Work out the finished part from the listing and answer in its coordinate system (mm). A direction names the side the tool comes from. Give positions to 0.01 mm unless a question says otherwise; leave off trailing zeros. Loops run counter-clockwise (first coordinate to the right, second up) from the corner with the lowest first, then second, coordinate; pieces in that order, holes last. Notation, with made-up numbers: (55, 26.5) - (71, 26.5) arc R26 cw to (71, 51.5) - close; hole circle Ø6 at (-35, -17). An arc over 180 degrees is marked (long way). Use one line per item in the form item = value. Start each with the question number.
Autodesk Inventor part; units mm, degrees
ref_plane "YZ Plane" through (0, 0, 0) normal (1, 0, 0) x (0, 1, 0)
ref_plane "XZ Plane" through (0, 0, 0) normal (0, 1, 0) x (-1, 0, 0)
ref_plane "XY Plane" through (0, 0, 0) normal (0, 0, 1) x (1, 0, 0)
sketch "Sketch1" plane through (0, 0, 0) normal (0, 1, 0) x (-1, 0, 0)
  circle A0 centre (0, 0) radius 21.5
  dimension "d0" = 43
extrude "Extrusion1" add sketch "Sketch1" along normal blind 68
sketch "Sketch2" plane through (0, 68, 0) normal (0, 1, 0) x (1, 0, 0)
  circle A0 centre (0, 0) radius 7.5
  dimension "d3" = 15
extrude "Extrusion2" add sketch "Sketch2" along normal blind 54
sketch "Sketch3" plane through (0, 0, 0) normal (0, -1, 0) x (1, 0, 0)
  line L0 (-15, 5) -> (-10, 5)
  line L1 (-10, 5) -> (-10, -5)
  line L2 (-10, -5) -> (-15, -5)
  line L3 (-15, -5) -> (-15, 5)
  line L4 (10, 5) -> (15, 5)
  line L5 (15, 5) -> (15, -5)
  line L6 (15, -5) -> (10, -5)
  line L7 (10, -5) -> (10, 5)
  line L8 (0, 0) -> (-29.5746, 0)
  circle A0 centre (0, 0) radius 7.5
  line L9 (0, 0) -> (0, 33.0968)
  dimension "d6" = 10
  dimension "d7" = 5
  dimension "d8" = 20
extrude "Extrusion3" add sketch "Sketch3" along normal blind 15 contours L0 L1 L8 L3 | L8 L1 L2 L3 | L4 L5 L6 L7
properties part number "Dremel motor"
1) A cutting plane is placed at B-B (z = 0). Give the vertices of the cut face in (x, y), plus the area to 3 significant figures.
2) A cutting plane is placed at D-D (x = 5.5). Give the vertices of the cut face in (y, z), plus the area to 3 significant figures.
3) Find the intervals of material crossed by probe 1 along X at (y, z) = (-4, -2); probe 2 along Y at (x, z) = (-17, 9.5); probe 3 along Z at (x, y) = (14, -4), in increasing order.
4) A cutting plane is placed at A-A (x = 0). Give the vertices of the cut face in (y, z), plus the area to 3 significant figures.
5) Flat-ended cylindrical pins translate along their axes: pin 1 Ø6 at (x, y) = (7.5, 20) entering from +Z; pin 2 Ø5 at (y, z) = (-11, 1) entering from +X; pin 3 Ø2.5 at (x, y) = (-13, -7) entering from +Z. Find the tip coordinate at first contact, or state that the pin passes through.
6) A cutting plane is placed at C-C (y = 42). Give the vertices of the cut face in (x, z), plus the area to 3 significant figures.
7) A tool of negligible diameter and unlimited length cuts with its end or side. For faces 4 (the cylindrical face through (-7.493, 94.622, 0.33)), 5 (the flat face through (-12, -7, -5)), 6 (the flat face through (12, -7, 5)), from which of +Z, -Z, +X, -X, +Y, -Y can it reach the whole face along a straight path? Write none if from no direction.
8) Determine the mould class of faces 1 (the cylindrical face through (2.799, 33.524, -21.317)), 2 (the flat face through (0, 0, 0)), 3 (the flat face through (-9, 68, 0)) for opening direction X: released by +X, released by -X, zero draft, split by the parting line, or undercut.
Answer sheet:
q1.outline = (-21.5, 0) - (-15, 0) - (-15, -15) - (-10, -15) - (-10, 0) - (10, 0) - (10, -15) - (15, -15) - (15, 0) - (21.5, 0) - (21.5, 68) - (7.5, 68) - (7.5, 122) - (-7.5, 122) - (-7.5, 68) - (-21.5, 68) - close
q1.area = 3,880 mm²
q2.outline = (0, -20.78) - (68, -20.78) - (68, -5.1) - (122, -5.1) - (122, 5.1) - (68, 5.1) - (68, 20.78) - (0, 20.78) - close
q2.area = 3,380 mm²
q3.probe_1 = -15 to -10, 10 to 15
q3.probe_2 = 0 to 68
q3.probe_3 = -5 to 5
q4.outline = (0, -21.5) - (68, -21.5) - (68, -7.5) - (122, -7.5) - (122, 7.5) - (68, 7.5) - (68, 21.5) - (0, 21.5) - close
q4.area = 3,730 mm²
q5.pin_1 = 21.02
q5.pin_2 = 15
q5.pin_3 = 5
q6.outline = circle Ø43 at (0, 0)
q6.area = 1,450 mm²
q7.face_4 = +Y
q7.face_5 = -Z, +X, -X, -Y
q7.face_6 = +Z, +X, -X, -Y
q8.face_1 = split by the parting line
q8.face_2 = undercut
q8.face_3 = zero draft
